Model file for the job. Use its own axes, mm. A direction names the side the tool comes from. Round coordinates to 2 decimals unless told otherwise and drop trailing zeros. Order: outer loops, then holes, each group sorted by start corner. A loop starts at its lowest first (then second) coordinate and runs counter-clockwise, first axis right, second up. Notation, with made-up numbers: (47, 1.25) - (75, 1.25) arc R11 cw to (75, 21.25) - close; hole circle Ø6 at (1.25, 55.5). An arc over 180 degrees is marked (long way). Use one line per item in the form item = value.
from build123d import *

# Parameters (mm, degrees)
F0_R      = 47.5
F0_R_2    = 35
F1_DEPTH  = 20
F0_W      = 120
F0_H      = 150
F0_R_3    = 8
F2_DEPTH  = 10
F2_FACE_R = 35
F3_DEPTH  = 10
F4_SIZE   = 5


with BuildPart() as f1:
    # F0 (on Front) → F1 (new body)
    with BuildSketch(Plane.XZ):
        Circle(F0_R)
        Circle(F0_R_2, mode=Mode.SUBTRACT)
    extrude(amount=F1_DEPTH)

    # F0 (on Front) → F2 (join)
    with BuildSketch(Plane.XZ):
        Rectangle(F0_W, F0_H)
        with Locations((-45, -60)):
            Circle(F0_R_3, mode=Mode.SUBTRACT)
        with Locations((45, -60)):
            Circle(F0_R_3, mode=Mode.SUBTRACT)
        with Locations((-45, 60)):
            Circle(F0_R_3, mode=Mode.SUBTRACT)
        Circle(F0_R, mode=Mode.SUBTRACT)
        with Locations((45, 60)):
            Circle(F0_R_3, mode=Mode.SUBTRACT)
        Circle(F0_R_2)
    extrude(amount=F2_DEPTH)

    # F2_face (on face) → F3 (join)
    with BuildSketch(Plane.XZ.offset(10)):
        Circle(F2_FACE_R)
    extrude(amount=F3_DEPTH)

    # F4
    f4_edges = [f1.edges().sort_by_distance(p)[0] for p in [
        (-60, -5, 75),
        (60, -5, 75),
        (60, -5, -75),
        (-60, -5, -75),
    ]]
    chamfer(f4_edges, length=F4_SIZE)


solid = f1.part
(1) Slice it at D-D on x = 45. Give the cut face in (y, z).
Report:
outline = (-20, -15.21) - (-10, -15.21) - (-10, -52) - (0, -52) - (0, 52) - (-10, 52) - (-10, 15.21) - (-20, 15.21) - close; (-10, -75) - (0, -75) - (0, -68) - (-10, -68) - close; (-10, 68) - (0, 68) - (0, 75) - (-10, 75) - close
(2) Slice it at A-A on y = -6.5. Give the cut face in (x, z).
Report:
outline = (-60, -70) - (-55, -75) - (55, -75) - (60, -70) - (60, 70) - (55, 75) - (-55, 75) - (-60, 70) - close; hole circle Ø16 at (-45, -60); hole circle Ø16 at (-45, 60); hole circle Ø16 at (45, -60); hole circle Ø16 at (45, 60)
(3) Pin check, flat tips, straight feed: pin 1 (4 mm diameter, centred on y = -14, z = -22, fed in from +X); pin 2 (18.5 mm diameter, centred on x = -45, z = 60, fed in from -Y). Stop position of each tip, or through.
Report:
pin_1 = 43.08
pin_2 = -10
(4) Tool access for faces 4 (the face through (-10.3, -14.93, -46.37)), 5 (the face through (-1, -20, 1)): list every direction of +Z, -Z, +X, -X, +Y, -Y with a clear straight run to the whole face (end or side of a thin tool).
Report:
face_4 = -Y
face_5 = +Z, -Z, +X, -X, -Y
(5) Slice it at C-C on x = 0. Give the cut face in (y, z), then the cut area to 3 significant figures.
Report:
outline = (-20, -47.5) - (-10, -47.5) - (-10, -75) - (0, -75) - (0, 75) - (-10, 75) - (-10, 47.5) - (-20, 47.5) - close
area = 2,450 mm2
(6) Probe probe 1 along Z at (x, y) = (-45, -5.5); probe 2 along Y at (x, z) = (45, -39); probe 3 along Z at (x, y) = (-17.5, -14.5). List the from-to ranges inside material, lowest first. Write a range as [from, to].
Report:
probe_1 = [-75, -68], [-52, 52], [68, 75]
probe_2 = [-10, 0]
probe_3 = [-44.16, 44.16]
(7) Pull direction X, two halves, no side cores. Call faces 1 (the face through (-46.041, -4.93, 67.932)), 2 (the face through (-57, -5, -73)), 3 (the face through (-1, -10, 51)): released by +X, released by -X, zero draft, split by the parting line, or undercut.
Report:
face_1 = undercut
face_2 = released by -X
face_3 = zero draft
(8) Slice it at B-B on z = -64. Give the cut face in (x, y).
Report:
outline = (-60, -10) - (-51.93, -10) - (-51.93, 0) - (-60, 0) - close; (-38.07, -10) - (38.07, -10) - (38.07, 0) - (-38.07, 0) - close; (51.93, -10) - (60, -10) - (60, 0) - (51.93, 0) - close
